Autodesk Inventor part; units mm, degrees
ref_plane "YZ Plane" through (0, 0, 0) normal (1, 0, 0) x (0, 1, 0)
ref_plane "XZ Plane" through (0, 0, 0) normal (0, 1, 0) x (-1, 0, 0)
ref_plane "XY Plane" through (0, 0, 0) normal (0, 0, 1) x (1, 0, 0)
sketch "Sketch1" plane through (0, 0, 0) normal (0, 1, 0) x (-1, 0, 0)
  circle A0 centre (0, 0) radius 20
  dimension "d0" = 40
extrude "Extrusion1" add sketch "Sketch1" along normal blind 2.6
sketch "Sketch2" plane through (0, 2.6, 0) normal (0, 1, 0) x (1, 0, 0)
  line L0 (-10, -10) -> (-10, 10)
  line L1 (-10, 10) -> (10, 10)
  line L2 (10, 10) -> (10, -10)
  line L3 (10, -10) -> (-10, -10)
  line L4 (-10, -10) -> (10, 10) construction
  line L5 (-10, 10) -> (10, -10) construction
  point P0 (0, 0)
  dimension "d3" = 20
  dimension "d4" = 20
extrude "Extrusion2" cut sketch "Sketch2" against normal blind 0.6
sketch "Sketch3" plane through (0, 2, 0) normal (0, 1, 0) x (1, 0, 0)
  line L0 (-6.8539, 8.6323) -> (6.8539, 8.6323) construction
  line L1 (6.8539, 8.6323) -> (6.8539, -8.5596) construction
  line L2 (6.8539, -8.5596) -> (-6.8539, -8.5596) construction
  line L3 (-6.8539, -8.5596) -> (-6.8539, 8.6323) construction
  spline S0 degree 2 poles (1.3116, -8.5596) (-0.3027, -8.5596) (-3.0335, -7.47) (-4.0289, -6.3803) knots 0 0 0 1 2 2 2
  spline S1 degree 2 poles (-4.0289, -6.3803) (-5.0244, -5.3042) (-6.114, -2.0756) (-6.114, 0.0229) knots 0 0 0 1 2 2 2
  spline S2 degree 2 poles (-6.114, 0.0229) (-6.114, 2.108) (-5.0513, 5.202) (-4.0424, 6.3454) knots 0 0 0 1 2 2 2
  spline S3 degree 2 poles (-4.0424, 6.3454) (-3.0469, 7.462) (-0.3296, 8.6323) (1.3519, 8.6323) knots 0 0 0 1 2 2 2
  spline S4 degree 2 poles (1.3519, 8.6323) (2.186, 8.6323) (3.6523, 8.3902) (4.2711, 8.2018) knots 0 0 0 1 2 2 2
  spline S5 degree 2 poles (4.2711, 8.2018) (4.8092, 8.027) (5.9257, 7.5292) (6.4772, 7.2333) knots 0 0 0 1 2 2 2
  line L4 (6.4772, 7.2333) -> (6.4772, 4.5697)
  line L5 (6.4772, 4.5697) -> (6.3024, 4.5697)
  spline S6 degree 2 poles (6.3024, 4.5697) (6.0064, 4.8388) (5.0917, 5.5921) (4.4325, 5.9553) knots 0 0 0 1 2 2 2
  spline S7 degree 2 poles (4.4325, 5.9553) (3.8002, 6.3051) (2.3071, 6.749) (1.3385, 6.749) knots 0 0 0 1 2 2 2
  spline S8 degree 2 poles (1.3385, 6.749) (0.2758, 6.749) (-1.621, 5.8746) (-2.334, 5.0406) knots 0 0 0 1 2 2 2
  spline S9 degree 2 poles (-2.334, 5.0406) (-3.0335, 4.1931) (-3.8137, 1.6237) (-3.8137, 0.0229) knots 0 0 0 1 2 2 2
  spline S10 degree 2 poles (-3.8137, 0.0229) (-3.8137, -1.6855) (-2.9931, -4.1473) (-2.2801, -4.9948) knots 0 0 0 1 2 2 2
  spline S11 degree 2 poles (-2.2801, -4.9948) (-1.5806, -5.8153) (0.2892, -6.6494) (1.3385, -6.6494) knots 0 0 0 1 2 2 2
  spline S12 degree 2 poles (1.3385, -6.6494) (2.2936, -6.6494) (3.9213, -6.1786) (4.5536, -5.8288) knots 0 0 0 1 2 2 2
  spline S13 degree 2 poles (4.5536, -5.8288) (5.1589, -5.479) (6.0602, -4.7526) (6.3158, -4.497) knots 0 0 0 1 2 2 2
  line L6 (6.3158, -4.497) -> (6.4772, -4.497)
  line L7 (6.4772, -4.497) -> (6.4772, -7.1337)
  spline S14 degree 2 poles (6.4772, -7.1337) (5.9257, -7.3893) (4.9571, -7.8601) (4.2711, -8.0753) knots 0 0 0 1 2 2 2
  spline S15 degree 2 poles (4.2711, -8.0753) (3.5447, -8.3175) (2.3071, -8.5596) (1.3116, -8.5596) knots 0 0 0 1 2 2 2
  point P0 (0, 0)
extrude "Extrusion3" add sketch "Sketch3" along normal blind 0.6
properties part number "TopMarkerPreset"
Model file for the job. Use its own axes, mm. Round coordinates to 2 decimals unless told otherwise and drop trailing zeros. Write each loop counter-clockwise with the first axis right and the second up, starting at its lowest first coordinate (ties: lowest second). Pieces come first, ordered by that corner, then holes. Notation, with made-up numbers: M 26,35.25 L 68,35.25 A24 ccw 68,74.25 Z; hole C 47,-22.75 d8. An arc over 180 degrees is marked long. Put each result on its own line as item: value.
Item 1: Cut at C-C (z = -16.5). List the corners of the cut face in (x, y), and give its area (3 significant figures).
Responses:
outline: M -11.3,0 L 11.3,0 L 11.3,2.6 L -11.3,2.6 Z
area: 58.8 mm²
Item 2: Cut at B-B (x = -8). List the corners of the cut face in (y, z), and give its area (3 significant figures).
Responses:
outline: M 0,-18.33 L 2.6,-18.33 L 2.6,-10 L 2,-10 L 2,10 L 2.6,10 L 2.6,18.33 L 0,18.33 Z
area: 83.3 mm²
Item 3: Cut at D-D (x = 9.5). List the corners of the cut face in (y, z).
Responses:
outline: M 0,-17.6 L 2.6,-17.6 L 2.6,-10 L 2,-10 L 2,10 L 2.6,10 L 2.6,17.6 L 0,17.6 Z
Item 4: Flat gauge pins, fed straight in: P1, Ø0.7, axis at y = 2.5, z = 5.5, coming from the +X side; P2, Ø1.5, axis at x = -11.5, y = 2, coming from the +Z side; P3, Ø0.5, axis at x = 5, y = 2.5, coming from the +Z side. Where does each tip first touch, or does it go through?
Responses:
P1: x = 19.33
P2: z = 16.87
P3: z = 19.43
Item 5: Mould opens along Z. For faces 1 (the flat face through (0, 2, 0)), 2 (the flat face through (-4, 2.6, 1)), 3 (the cylindrical face through (4.336, 1.282, 19.524)) say: +Z half, -Z half, draft (parallel to the pull), parting line (faces both ways), or undercut.
Responses:
face 1: undercut
face 2: draft
face 3: parting line
Item 6: Cut at A-A (y = 1.1). List the corners of the cut face in (x, z).
Responses:
outline: C 0,0 d40
Item 7: Probe L1, parallel to X at y = 2.25, z = 1.5; L2, parallel to X at y = 2.35, z = -2; L3, parallel to Y at x = -7.5, z = 5. List the from-to ranges inside material, lowest first. Write a range as from..to.
Responses:
L1: -19.94..-10, -6.04..-3.72, 10..19.94
L2: -19.9..-10, -5.98..-3.64, 10..19.9
L3: 0..2
